The model under review builds one solid part; all positions refer to its coordinate system, in mm. A direction names the side the tool comes from. Coordinates: 2 decimals unless noted, no trailing zeros. Order: outer loops, then holes, each group sorted by start corner. A loop starts at its lowest first (then second) coordinate and runs counter-clockwise, first axis right, second up. Notation, with made-up numbers: (52.25, 68.25) -> (105.25, 68.25) arc R19 ccw to (105.25, 85.25) -> close; hole circle Ø4 at (28.25, -1.5). An arc over 180 degrees is marked (long way). Use one line per item in the form item = value.
from build123d import *

# Parameters (mm, degrees)
SKETCH_1_R      = 1.6
SKETCH_1_R_2    = 8
EXTRUDE_1_DEPTH = 14.5


with BuildPart() as part:
    # 草图1 → 凸台-拉伸1 (new body)
    with BuildSketch(Plane(origin=(0, 7.25, 0), x_dir=(1, 0, 0), z_dir=(0, 1, 0))):
        with BuildLine():
            Line((10.270859413, -14.168960686), (18.367408376, -8.299898164))
            ThreePointArc((18.367408376, -8.299898164), (22.961692064, 13.256939094), (1.995781529, 20.056591338))
            Line((1.995781529, 20.056591338), (-7.135250193, 15.979305513))
            ThreePointArc((-7.135250193, 15.979305513), (-15.155444566, -8.75), (10.270859413, -14.168960686))
        make_face()
        with Locations((-11.691342951, -6.75)):
            Circle(SKETCH_1_R, mode=Mode.SUBTRACT)
        with Locations((-11.691342951, 6.75)):
            Circle(SKETCH_1_R, mode=Mode.SUBTRACT)
        with Locations((0, 13.5)):
            Circle(SKETCH_1_R, mode=Mode.SUBTRACT)
        with Locations((11.691342951, 6.75)):
            Circle(SKETCH_1_R, mode=Mode.SUBTRACT)
        with Locations((11.691342951, -6.75)):
            Circle(SKETCH_1_R, mode=Mode.SUBTRACT)
        with Locations((0, -13.5)):
            Circle(SKETCH_1_R, mode=Mode.SUBTRACT)
        Circle(SKETCH_1_R_2, mode=Mode.SUBTRACT)
        with BuildLine():
            Line((18.998716884, -0.241336031), (18.958263766, -0.241336031))
            ThreePointArc((18.958263766, -0.241336031), (17.933337503, 0.163435155), (17.461558732, 1.159295761))
            ThreePointArc((17.461558732, 1.159295761), (15.155444566, 8.75), (9.734758946, 14.542505571))
            ThreePointArc((9.734758946, 14.542505571), (9.108207748, 15.449008275), (9.27012875, 16.539006048))
            Line((9.27012875, 16.539006048), (9.290355309, 16.574039476))
            ThreePointArc((9.290355309, 16.574039476), (9.954159898, 17.182891337), (10.847026058, 17.301748995))
            ThreePointArc((10.847026058, 17.301748995), (19.497590449, 11.256939094), (20.407267188, 0.742925624))
            ThreePointArc((20.407267188, 0.742925624), (19.857900358, 0.029109677), (18.998716884, -0.241336031))
        make_face(mode=Mode.SUBTRACT)
        with BuildLine():
            ThreePointArc((4.813837212, -9.890751807), (5.5, -9.526279442), (6.158723721, -9.114281218))
            ThreePointArc((6.158723721, -9.114281218), (8.588519962, -9.584483547), (8.118317632, -12.014279788))
            ThreePointArc((8.118317632, -12.014279788), (7.25, -12.557368355), (6.345512688, -13.0378092))
            ThreePointArc((6.345512688, -13.0378092), (4.006146253, -12.230118241), (4.813837212, -9.890751807))
        make_face(mode=Mode.SUBTRACT)
        with BuildLine():
            ThreePointArc((-6.158723721, -9.114281218), (-5.5, -9.526279442), (-4.813837212, -9.890751807))
            ThreePointArc((-4.813837212, -9.890751807), (-4.006146253, -12.230118241), (-6.345512688, -13.0378092))
            ThreePointArc((-6.345512688, -13.0378092), (-7.25, -12.557368355), (-8.118317632, -12.014279788))
            ThreePointArc((-8.118317632, -12.014279788), (-8.588519962, -9.584483547), (-6.158723721, -9.114281218))
        make_face(mode=Mode.SUBTRACT)
        with BuildLine():
            ThreePointArc((-10.972560933, 0.776470588), (-11, 0), (-10.972560933, -0.776470588))
            ThreePointArc((-10.972560933, -0.776470588), (-12.594666215, -2.645634694), (-14.463830321, -1.023529412))
            ThreePointArc((-14.463830321, -1.023529412), (-14.5, 0), (-14.463830321, 1.023529412))
            ThreePointArc((-14.463830321, 1.023529412), (-12.594666215, 2.645634694), (-10.972560933, 0.776470588))
        make_face(mode=Mode.SUBTRACT)
        with BuildLine():
            ThreePointArc((-4.813837212, 9.890751807), (-5.5, 9.526279442), (-6.158723721, 9.114281218))
            ThreePointArc((-6.158723721, 9.114281218), (-8.588519962, 9.584483547), (-8.118317632, 12.014279788))
            ThreePointArc((-8.118317632, 12.014279788), (-7.25, 12.557368355), (-6.345512688, 13.0378092))
            ThreePointArc((-6.345512688, 13.0378092), (-4.006146253, 12.230118241), (-4.813837212, 9.890751807))
        make_face(mode=Mode.SUBTRACT)
        with BuildLine():
            ThreePointArc((6.158723721, 9.114281218), (5.5, 9.526279442), (4.813837212, 9.890751807))
            ThreePointArc((4.813837212, 9.890751807), (4.006146253, 12.230118241), (6.345512688, 13.0378092))
            ThreePointArc((6.345512688, 13.0378092), (7.25, 12.557368355), (8.118317632, 12.014279788))
            ThreePointArc((8.118317632, 12.014279788), (8.588519962, 9.584483547), (6.158723721, 9.114281218))
        make_face(mode=Mode.SUBTRACT)
        with BuildLine():
            ThreePointArc((10.972560933, -0.776470588), (11, 0), (10.972560933, 0.776470588))
            ThreePointArc((10.972560933, 0.776470588), (12.594666215, 2.645634694), (14.463830321, 1.023529412))
            ThreePointArc((14.463830321, 1.023529412), (14.5, 0), (14.463830321, -1.023529412))
            ThreePointArc((14.463830321, -1.023529412), (12.594666215, -2.645634694), (10.972560933, -0.776470588))
        make_face(mode=Mode.SUBTRACT)
    extrude(amount=-EXTRUDE_1_DEPTH)


solid = part.part
Item 1: To check wall thickness, follow L1, parallel to Z at x = 11.5, y = -2; L2, parallel to X at y = -3.25, z = -6.75; L3, parallel to X at y = 0.75, z = -9. State the ranges of each line that lie inside material, in increasing order. Write a range as from..to.
Results found:
L1 = -21.25..-17.17, -13.19..-8.34, -5.16..-2.16, 2.16..5.16, 8.34..13.28
L2 = -16.15..-13.29, -10.09..-4.29, 4.29..10.09, 13.29..16.15, 21.05..25.08
L3 = -15.01..-7.92, -6.35..6.35, 7.92..15.01, 20.52..24.68
Item 2: Tool access review of faces 4 (the face through (8, 7.25, -2)), 5 (the face through (7.238, 0.101, -12.565)): name each direction out of +Z, -Z, +X, -X, +Y, -Y from which nothing blocks a thin tool from reaching the whole face with its end or side.
Results found:
face_4 = +Z, -Z, +X, -X, +Y
face_5 = +Y, -Y
Item 3: Draft analysis for pull direction Z (two halves, no side actions). For faces 1 (the face through (23.13, 0.1, -12.96)), 2 (the face through (14.262, 0.101, 11.276)), 3 (the face through (-11, 0, 0)), state which applies: released by +Z, released by -Z, zero draft, split by the parting line, or undercut.
Results found:
face_1 = split by the parting line
face_2 = released by +Z
face_3 = undercut
Item 4: We need section A-A (x = 3). Write out the cut boundary in (y, z), plus the area to 3 significant figures.
Results found:
outline = (-7.25, -20.47) -> (7.25, -20.47) -> (7.25, -7.42) -> (-7.25, -7.42) -> close; (-7.25, 7.42) -> (7.25, 7.42) -> (7.25, 17.24) -> (-7.25, 17.24) -> close
area = 332 mm²
Item 5: We need section B-B (z = -6.75). Write out the cut boundary in (x, y).
Results found:
outline = (-16.15, -7.25) -> (-13.29, -7.25) -> (-13.29, 7.25) -> (-16.15, 7.25) -> close; (-10.09, -7.25) -> (-4.29, -7.25) -> (-4.29, 7.25) -> (-10.09, 7.25) -> close; (4.29, -7.25) -> (10.09, -7.25) -> (10.09, 7.25) -> (4.29, 7.25) -> close; (13.29, -7.25) -> (16.15, -7.25) -> (16.15, 7.25) -> (13.29, 7.25) -> close; (21.05, -7.25) -> (25.08, -7.25) -> (25.08, 7.25) -> (21.05, 7.25) -> close
Item 6: We need section C-C (y = 1.75). State how many separate pieces and enclosed holes the cut face has, plus the area to 3 significant figures.
Results found:
separate_pieces = 1
enclosed_holes = 14
area = 819 mm²
Item 7: Clearance check with flat-ended pins moving along their axes: pin 1 (3 mm diameter, centred on y = -5, z = -7, fed in from +X); pin 2 (1.9 mm diameter, centred on x = -11.69, z = -6.75, fed in from +Y); pin 3 (1.5 mm diameter, centred on y = -2.5, z = -3, fed in from +X); pin 4 (4 mm diameter, centred on y = 2.5, z = -16.5, fed in from -X). State where each tip first meets the part, or that it passes through.
Results found:
pin_1 = 25.16
pin_2 = through
pin_3 = 25.12
pin_4 = -9.8
